from build123d import *

# Parameters (mm, degrees)
SKETCH1_R           = 19.05
BOSS_EXTRUDE1_DEPTH = 50.8
SKETCH2_R           = 4.0000047
CUT_EXTRUDE1_DEPTH  = 25.4
SKETCH4_R           = 4
SKETCH4_R_2         = 2
CUT_EXTRUDE2_DEPTH  = 25.4
SKETCH6_R           = 2
CUT_EXTRUDE3_DEPTH  = 12.7
SKETCH7_R           = 19.05
CUT_EXTRUDE4_DEPTH  = 6.35


with BuildPart() as part:
    # Sketch1 → Boss-Extrude1 (new body)
    with BuildSketch(Plane(origin=(0, 0, 0), x_dir=(1, 0, 0), z_dir=(0, 1, 0))):
        Circle(SKETCH1_R)
    extrude(amount=BOSS_EXTRUDE1_DEPTH)

    # Sketch2 → Cut-Extrude1 (cut)
    with BuildSketch(Plane(origin=(0, 50.8, 0), x_dir=(1, 0, 0), z_dir=(0, 1, 0))):
        Circle(SKETCH2_R)
    extrude(amount=-CUT_EXTRUDE1_DEPTH, mode=Mode.SUBTRACT)

    # Sketch4 → Cut-Extrude2 (cut)
    with BuildSketch(Plane(origin=(0, 0, -19.05), x_dir=(-1, 0, 0), z_dir=(0, 0, -1))):
        with Locations((0, 12.7)):
            Circle(SKETCH4_R)
        with Locations((0.188503161, 38.1)):
            Circle(SKETCH4_R_2)
    extrude(amount=-CUT_EXTRUDE2_DEPTH, mode=Mode.SUBTRACT)

    # Sketch6 → Cut-Extrude3 (cut)
    with BuildSketch(Plane.XZ):
        Circle(SKETCH6_R)
    extrude(amount=-CUT_EXTRUDE3_DEPTH, mode=Mode.SUBTRACT)

    # Sketch7 → Cut-Extrude4 (cut)
    with BuildSketch(Plane(origin=(0, 50.8, 0), x_dir=(1, 0, 0), z_dir=(0, 1, 0))):
        Circle(SKETCH7_R)
    extrude(amount=-CUT_EXTRUDE4_DEPTH, mode=Mode.SUBTRACT)


solid = part.part
Geometry: final body of the model. Coordinates: model frame, mm. A direction names the side the tool comes from. Give positions to 0.01 mm unless a question says otherwise; leave off trailing zeros. Write each loop counter-clockwise with the first axis right and the second up, starting at its lowest first coordinate (ties: lowest second). Pieces come first, ordered by that corner, then holes.
(1) First-contact query: P1, Ø3, axis at y = 18.5, z = -14, coming from the +X side; P2, Ø12, axis at x = -8.5, y = 13, coming from the -Z side; P3, Ø10.5, axis at x = 0, y = 12.7, coming from the +Z side. Flat tips, straight axial feed; report the tip coordinate or a pass-through.
(2) Ray query, line 1 (Y direction, x = 0, z = -16.5); line 2 (X direction, y = 5.75, z = 0); line 3 (Y direction, x = -1, z = -13.5). Return the intervals inside material, ascending.
(3) Cut plane B-B, the plane x = 0.5. Return loops of the section in (y, z).
(4) Access query for faces 4 (the cylindrical face through (0, 5, -2)), 5 (the cylindrical face through (-4.13, 21.914, 18.597)), 6 (the cylindrical face through (3.815, 35.058, -1.201)), 7 (the flat face through (0, 44.45, -5)), 8 (the flat face through (0, 13, 6.35)). Directions: +Z, -Z, +X, -X, +Y, -Y. A direction counts if a zero-diameter tool reaches every point of the face in a straight line with its end or side. Return the directions, or none.
(5) Cut plane A-A, the plane y = 6. Return loops of the section in (x, z), then the cut area to 3 significant figures.
(6) Cut plane D-D, the plane y = 38.1. Return loops of the section in (x, z), then the cut area to 3 significant figures.
(7) Cut plane C-C, the plane z = 0. Return loops of the section in (x, y), then the cut area to 3 significant figures.
(8) Mould query, pull axis Y, two halves, no side actions, for faces 1 (the flat face through (4, 0, 0)), 2 (the flat face through (0, 25.4, 0)), 3 (the flat face through (0, 38, 6.35)). Classes: released by +Y, released by -Y, zero draft, split by the parting line, or undercut.
Values follow:
1. P1: stops at x = 14.38
1. P2: stops at z = -18.81
1. P3: stops at z = 19.05
2. line 1: y = 0 to 8.7, 16.7 to 36.11, 40.09 to 44.45
2. line 2: x = -19.05 to -2, 2 to 19.05
2. line 3: y = 0 to 8.83, 16.57 to 36.27, 39.93 to 44.45
3. outline: (0, -19.04) - (8.73, -19.04) - (8.73, -1.94) - (0, -1.94) - close; (0, 1.94) - (8.73, 1.94) - (8.73, 6.35) - (16.67, 6.35) - (16.67, -19.04) - (36.22, -19.04) - (36.22, -3.97) - (25.4, -3.97) - (25.4, 3.97) - (36.22, 3.97) - (36.22, 6.35) - (39.98, 6.35) - (39.98, 3.97) - (44.45, 3.97) - (44.45, 19.04) - (0, 19.04) - close; (39.98, -19.04) - (44.45, -19.04) - (44.45, -3.97) - (39.98, -3.97) - close
4. face 4: -Y
4. face 5: +Y, -Y
4. face 6: +Y
4. face 7: +Z, -Z, +X, -X, +Y
4. face 8: -Z
5. outline: circle Ø38.1 at (0, 0); hole circle Ø4 at (0, 0)
5. area: 1,130 mm2
6. outline: (-2.19, -18.92) - (-2.19, -3.35) arc R4 cw to (-2.19, 3.35) - (-2.19, 6.35) - (1.81, 6.35) - (1.81, 3.57) arc R4 cw to (1.81, -3.57) - (1.81, -18.96) arc R19.05 ccw (long way) to start
6. area: 1,020 mm2
7. outline: (-19.05, 0) - (-2, 0) - (-2, 9.24) arc R4 cw (long way) to (2, 9.24) - (2, 0) - (19.05, 0) - (19.05, 44.45) - (4, 44.45) - (4, 25.4) - (-4, 25.4) - (-4, 44.45) - (-19.05, 44.45) - close
7. area: 1,460 mm2
8. face 1: released by -Y
8. face 2: released by +Y
8. face 3: undercut
